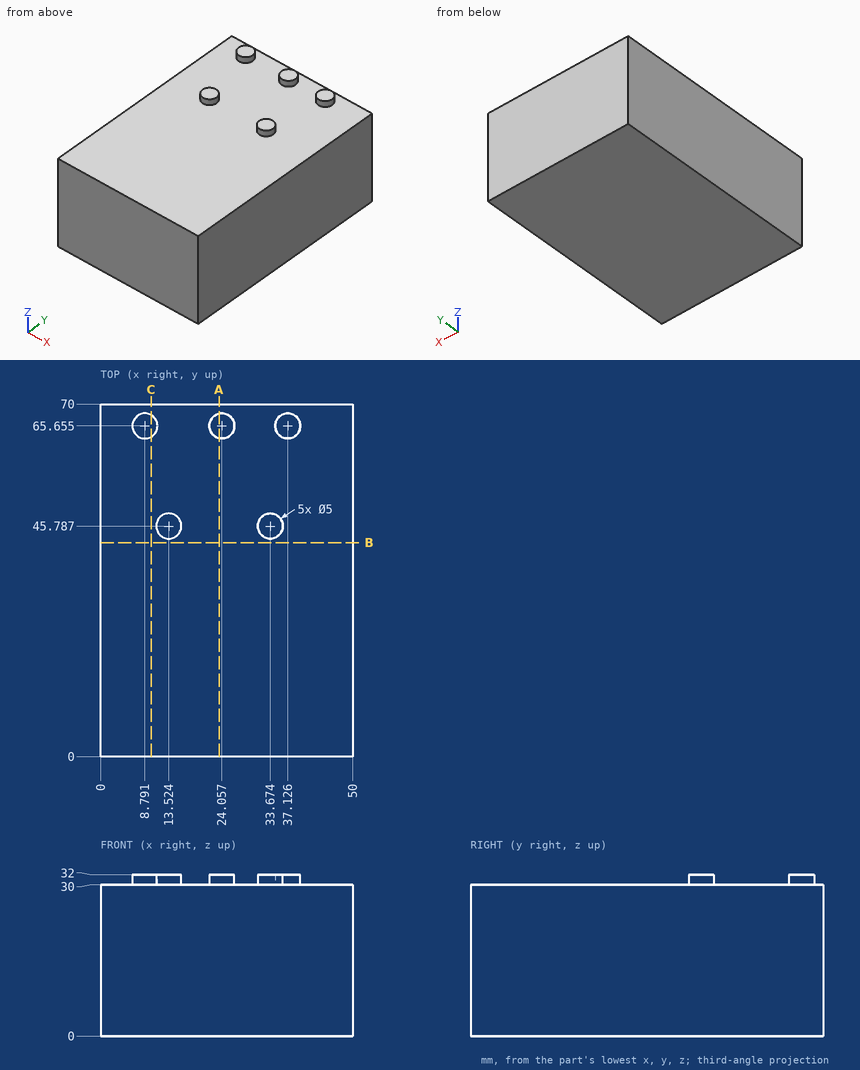
Could you check a few things on this drawing? It's one solid part, dimensions in mm from its lowest x, y, z. Give positions to 0.01 mm unless a question says otherwise; leave off trailing zeros. Order: outer loops, then holes, each group sorted by start corner. A loop starts at its lowest first (then second) coordinate and runs counter-clockwise, first axis right, second up. Notation, with made-up numbers: (24, -38) - (48, -38) arc R35 ccw to (48, 1) - close; hole circle Ø8 at (87, 9.5). An arc over 180 degrees is marked (long way). Answer as a JSON object with one key per item and string values. Group by question number.
Item 1: If we section it at A-A on x = 23.5: Please give me the cut outline in (y, z).
Item 2: Please list where this line runs through material, in increasing order: probe 1 along Z at (x, y) = (38.5, 6).
Item 3: If we section it at B-B on y = 42.5: Please give me the cut outline in (x, z), and give its area (3 significant figures).
Item 4: If we section it at C-C on x = 10: Please give me the cut outline in (y, z), and give its area (3 significant figures).
Result set:
{
 "1": {"outline": "(0, 0) - (70, 0) - (70, 30) - (68.09, 30) - (68.09, 32) - (63.22, 32) - (63.22, 30) - (0, 30) - close"},
 "2": {"probe 1": "0 to 30"},
 "3": {"outline": "(0, 0) - (50, 0) - (50, 30) - (0, 30) - close", "area": "1,500 mm²"},
 "4": {"outline": "(0, 0) - (70, 0) - (70, 30) - (67.84, 30) - (67.84, 32) - (63.47, 32) - (63.47, 30) - (0, 30) - close", "area": "2,110 mm²"}
}
